For this review, take the finished solid that the model builds, in its own axes (mm). Face numbers are marked on the shaded views. A direction names the side the tool comes from. Coordinates: 2 decimals unless noted, no trailing zeros. Loops run counter-clockwise (first coordinate to the right, second up) from the corner with the lowest first, then second, coordinate; pieces in that order, holes last. Notation, with made-up numbers: (-24.5, 20) -> (-13.5, 20) arc R28 cw to (-13.5, 52) -> close; hole circle Ø2 at (30.5, -21). An arc over 180 degrees is marked (long way). Use a Markdown table: item, result.
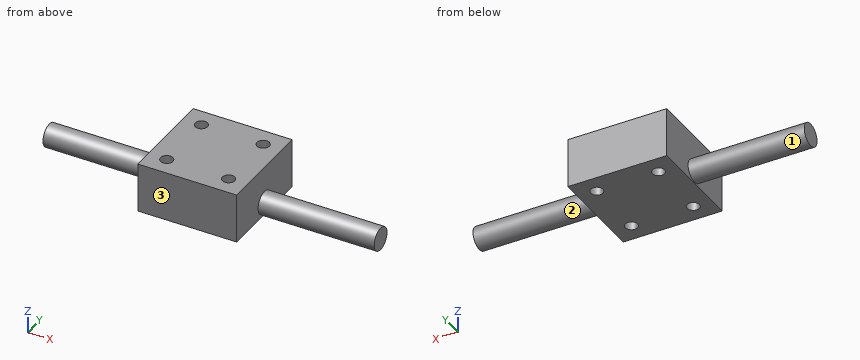
from build123d import *

# Parameters (mm, degrees)
F0_W     = 50.8
F0_H     = 50.8
F0_R     = 3.175
F1_DEPTH = 12.7
F2_R     = 5.851263
F3_DEPTH = 85.09


with BuildPart() as f1:
    # F0 (on Top) → F1 (new body, symmetric)
    with BuildSketch(Plane.XY):
        Rectangle(F0_W, F0_H)
        with Locations((-15.875, -15.875)):
            Circle(F0_R, mode=Mode.SUBTRACT)
        with Locations((15.875, -15.875)):
            Circle(F0_R, mode=Mode.SUBTRACT)
        with Locations((-15.875, 15.875)):
            Circle(F0_R, mode=Mode.SUBTRACT)
        with Locations((15.875, 15.875)):
            Circle(F0_R, mode=Mode.SUBTRACT)
    extrude(amount=F1_DEPTH, both=True)

    # F2 (on Right) → F3 (join)
    with BuildSketch(Plane.YZ):
        with Locations((0, -6.202326)):
            Circle(F2_R)
    extrude(amount=F3_DEPTH)

    # F4: F1 across plane


with BuildPart() as f1_1:
    add(f1.part)
    add(f1.part.mirror(Plane.YZ))


solid = f1_1.part
(1) Take a section at D-D on z = 4.25. Write out the cut boundary in (x, y) (3 decimals), plus the area to 3 significant figures.
Found:
| item | result |
|---|---|
| outline | (-25.4, -25.4) -> (25.4, -25.4) -> (25.4, 25.4) -> (-25.4, 25.4) -> close; hole circle Ø6.35 at (-15.875, -15.875); hole circle Ø6.35 at (-15.875, 15.875); hole circle Ø6.35 at (15.875, -15.875); hole circle Ø6.35 at (15.875, 15.875) |
| area | 2,450 mm^2 |
(2) Take a section at C-C on x = 17. Write out the cut boundary in (y, z).
Found:
| item | result |
|---|---|
| outline | (-25.4, -12.7) -> (-18.84, -12.7) -> (-18.84, 12.7) -> (-25.4, 12.7) -> close; (-12.91, -12.7) -> (12.91, -12.7) -> (12.91, 12.7) -> (-12.91, 12.7) -> close; (18.84, -12.7) -> (25.4, -12.7) -> (25.4, 12.7) -> (18.84, 12.7) -> close |
(3) For line 1 along Y through (x, z) = (-16.5, -1.25); line 2 along X through (y, z) = (11, 4.75); line 3 along Z through (x, y) = (-60.5, -1), list the stretches that pass through material, from the lowest coordinate up.
Found:
| item | result |
|---|---|
| line 1 | y = -25.4 to -18.99, -12.76 to 12.76, 18.99 to 25.4 |
| line 2 | x = -25.4 to 25.4 |
| line 3 | z = -11.97 to -0.44 |
(4) Take a section at B-B on z = -2.25. Write out the cut boundary in (x, y) (3 decimals), plus the area to 3 significant figures.
Found:
| item | result |
|---|---|
| outline | (-85.09, -4.315) -> (-25.4, -4.315) -> (-25.4, -25.4) -> (25.4, -25.4) -> (25.4, -4.315) -> (85.09, -4.315) -> (85.09, 4.315) -> (25.4, 4.315) -> (25.4, 25.4) -> (-25.4, 25.4) -> (-25.4, 4.315) -> (-85.09, 4.315) -> close; hole circle Ø6.35 at (-15.875, -15.875); hole circle Ø6.35 at (-15.875, 15.875); hole circle Ø6.35 at (15.875, -15.875); hole circle Ø6.35 at (15.875, 15.875) |
| area | 3,480 mm^2 |
(5) For the marked faces 1, 2 and 3, list the 3-axis set-ups (+Z, -Z, +X, -X, +Y, -Y) from which the entire face can be reached by the end or side of a thin tool; tool diameter is ignored.
Found:
| item | result |
|---|---|
| face 1 | -X |
| face 2 | +X |
| face 3 | +Z, -Z, +X, -X, -Y |
(6) For pin 1 Ø4 at (y, z) = (10.5, -6) entering from -X; pin 2 Ø4 at (x, y) = (-15.875, 15.875) entering from -Z (1 decimal); pin 3 Ø1 at (x, z) = (64, -6) entering from +Y; pin 4 Ø6 at (y, z) = (5, 3) entering from +X, all flat-tipped, find the tip position at first contact; note any pin that passes through.
Found:
| item | result |
|---|---|
| pin 1 | stops at x = -25.4 |
| pin 2 | passes through |
| pin 3 | stops at y = 5.85 |
| pin 4 | stops at x = 25.4 |
(7) Take a section at A-A on y = 0. Write out the cut boundary in (x, z), plus the area to 3 significant figures.
Found:
| item | result |
|---|---|
| outline | (-85.09, -12.05) -> (-25.4, -12.05) -> (-25.4, -12.7) -> (25.4, -12.7) -> (25.4, -12.05) -> (85.09, -12.05) -> (85.09, -0.35) -> (25.4, -0.35) -> (25.4, 12.7) -> (-25.4, 12.7) -> (-25.4, -0.35) -> (-85.09, -0.35) -> close |
| area | 2,690 mm^2 |
